Design review of the part built by this model. Coordinates are the model's own, in mm. Face numbers are marked on the shaded views. A direction names the side the tool comes from. Coordinates: 2 decimals unless noted, no trailing zeros. Order: outer loops, then holes, each group sorted by start corner. A loop starts at its lowest first (then second) coordinate and runs counter-clockwise, first axis right, second up. Notation, with made-up numbers: M 81.5,10.25 L 125.5,10.25 A15 ccw 125.5,37.25 Z; hole C 5,69.5 d11. An arc over 180 degrees is marked long. Use CSV: the item, a comma, the result in double quotes.
```python
from build123d import *

# Parameters (mm, degrees)
F0_R     = 3.5
F0_W     = 22
F0_H     = 15
F1_DEPTH = 2
F2_DEPTH = 25
F3_DEPTH = 2


with BuildPart() as f1:
    # F0 (on Top) → F1 (new body)
    with BuildSketch(Plane.XY):
        with BuildLine():
            Line((-23.506553, -5.771502), (-6.866502, -10.5))
            Line((-6.866502, -10.5), (51.133498, -10.5))
            ThreePointArc((51.133498, -10.5), (52.358243, -10.081139), (53.06999, -9))
            ThreePointArc((53.06999, -9), (53.117558, -8.752009), (53.133498, -8.5))
            Line((53.133498, -8.5), (53.133498, 8.5))
            ThreePointArc((53.133498, 8.5), (53.117558, 8.752009), (53.06999, 9))
            ThreePointArc((53.06999, 9), (52.358243, 10.081139), (51.133498, 10.5))
            Line((51.133498, 10.5), (-6.866502, 10.5))
            Line((-6.866502, 10.5), (-23.506553, 5.771502))
            ThreePointArc((-23.506553, 5.771502), (-27.866502, 0), (-23.506553, -5.771502))
        make_face()
        with Locations((-21.866502, 0)):
            Circle(F0_R, mode=Mode.SUBTRACT)
        with Locations((4.133498, 0)):
            Rectangle(F0_W, F0_H, mode=Mode.SUBTRACT)
        with BuildLine():
            ThreePointArc((17.881379, -9), (16.820718, -8.56066), (16.381379, -7.5))
            Line((16.381379, -7.5), (16.381379, 7.5))
            ThreePointArc((16.381379, 7.5), (16.820718, 8.56066), (17.881379, 9))
            Line((17.881379, 9), (51.133498, 9))
            ThreePointArc((51.133498, 9), (52.194158, 8.56066), (52.633498, 7.5))
            Line((52.633498, 7.5), (52.633498, -7.5))
            ThreePointArc((52.633498, -7.5), (52.194158, -8.56066), (51.133498, -9))
            Line((51.133498, -9), (17.881379, -9))
        make_face(mode=Mode.SUBTRACT)
    extrude(amount=F1_DEPTH)

    # F0 (on Top) → F2 (join)
    with BuildSketch(Plane.XY):
        with BuildLine():
            Line((16.381379, 7.5), (16.381379, -7.5))
            ThreePointArc((16.381379, -7.5), (16.820718, -8.56066), (17.881379, -9))
            Line((17.881379, -9), (51.133498, -9))
            ThreePointArc((51.133498, -9), (52.194158, -8.56066), (52.633498, -7.5))
            Line((52.633498, -7.5), (52.633498, 7.5))
            ThreePointArc((52.633498, 7.5), (52.194158, 8.56066), (51.133498, 9))
            Line((51.133498, 9), (17.881379, 9))
            ThreePointArc((17.881379, 9), (16.820718, 8.56066), (16.381379, 7.5))
        make_face()
        with BuildLine():
            Line((49.633498, -7.5), (19.381379, -7.5))
            ThreePointArc((19.381379, -7.5), (18.320718, -7.06066), (17.881379, -6))
            Line((17.881379, -6), (17.881379, 6))
            ThreePointArc((17.881379, 6), (18.320718, 7.06066), (19.381379, 7.5))
            Line((19.381379, 7.5), (49.633498, 7.5))
            ThreePointArc((49.633498, 7.5), (50.694158, 7.06066), (51.133498, 6))
            Line((51.133498, 6), (51.133498, -6))
            ThreePointArc((51.133498, -6), (50.694158, -7.06066), (49.633498, -7.5))
        make_face(mode=Mode.SUBTRACT)
    extrude(amount=F2_DEPTH)

    # F0 (on Top) → F3 (join)
    with BuildSketch(Plane.XY):
        with BuildLine():
            ThreePointArc((17.881379, -6), (18.320718, -7.06066), (19.381379, -7.5))
            Line((19.381379, -7.5), (49.633498, -7.5))
            ThreePointArc((49.633498, -7.5), (50.694158, -7.06066), (51.133498, -6))
            Line((51.133498, -6), (51.133498, 6))
            ThreePointArc((51.133498, 6), (50.694158, 7.06066), (49.633498, 7.5))
            Line((49.633498, 7.5), (19.381379, 7.5))
            ThreePointArc((19.381379, 7.5), (18.320718, 7.06066), (17.881379, 6))
            Line((17.881379, 6), (17.881379, -6))
        make_face()
    extrude(amount=F3_DEPTH)


solid = f1.part
```
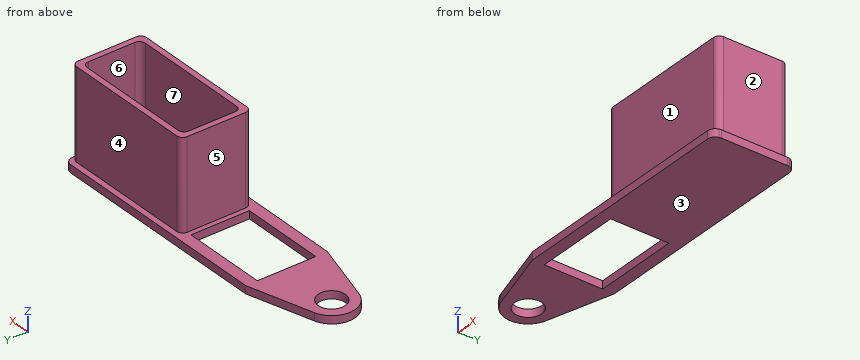
(1) Clearance check with flat-ended pins moving along their axes: P1, Ø0.6, axis at y = 3.5, z = 1.5, coming from the -X side; P2, Ø8, axis at y = 7.5, z = 10.5, coming from the -X side; P3, Ø1, axis at y = 8, z = 15.5, coming from the +X side. State where each tip first meets the part, or that it passes through.
The answers:
P1,"stops at x = -26.94"
P2,"stops at x = 16.38"
P3,"stops at x = 52.63"
(2) Add section A-A on y = 0. State the section outline as (x, z) points.
The answers:
outline,"M -27.87,0 L -25.37,0 L -25.37,2 L -27.87,2 Z; M -18.37,0 L -6.87,0 L -6.87,2 L -18.37,2 Z; M 15.13,0 L 53.13,0 L 53.13,2 L 52.63,2 L 52.63,25 L 51.13,25 L 51.13,2 L 17.88,2 L 17.88,25 L 16.38,25 L 16.38,2 L 15.13,2 Z"
(3) Wall thickness on probe 1 along Y at (x, z) = (23.5, 19); probe 2 along X at (y, z) = (-5.5, 4); probe 3 along Z at (x, y) = (18.5, 4.25): over which ranges is each line inside the solid? List them lowest first.
The answers:
probe 1,"y = -9 to -7.5, 7.5 to 9"
probe 2,"x = 16.38 to 17.88, 51.13 to 52.63"
probe 3,"z = 0 to 2"
(4) For the marked faces 1, 2 and 3, list the 3-axis set-ups (+Z, -Z, +X, -X, +Y, -Y) from which the entire face can be reached by the end or side of a thin tool; tool diameter is ignored.
The answers:
face 1,"+Z, +X, -X, -Y"
face 2,"+Z, +X, +Y, -Y"
face 3,"-Z, +X, -X, +Y, -Y"
(5) Add section D-D on x = 48. State the section outline as (y, z) points, and give its area (3 significant figures).
The answers:
outline,"M -10.5,0 L 10.5,0 L 10.5,2 L 9,2 L 9,25 L 7.5,25 L 7.5,2 L -7.5,2 L -7.5,25 L -9,25 L -9,2 L -10.5,2 Z"
area,"111 mm2"
(6) The part is to be moulded in two halves that separate along X. For the marked faces 4, 5, 6 and 7, say which applies: pulls with the +X half, pulls with the -X half, needs draft (parallel to the pull), parting line crosses it, or undercut.
The answers:
face 4,"needs draft"
face 5,"pulls with the -X half"
face 6,"undercut"
face 7,"undercut"
(7) Add section B-B on x = -5. State the section outline as (y, z) points.
The answers:
outline,"M -10.5,0 L -7.5,0 L -7.5,2 L -10.5,2 Z; M 7.5,0 L 10.5,0 L 10.5,2 L 7.5,2 Z"
(8) Add section C-C on z = 20.5. State the section outline as (x, y) points.
The answers:
outline,"M 16.38,-7.5 A1.5 ccw 17.88,-9 L 51.13,-9 A1.5 ccw 52.63,-7.5 L 52.63,7.5 A1.5 ccw 51.13,9 L 17.88,9 A1.5 ccw 16.38,7.5 Z; hole M 17.88,-6 A1.5 ccw 19.38,-7.5 L 49.63,-7.5 A1.5 ccw 51.13,-6 L 51.13,6 A1.5 ccw 49.63,7.5 L 19.38,7.5 A1.5 ccw 17.88,6 Z"
